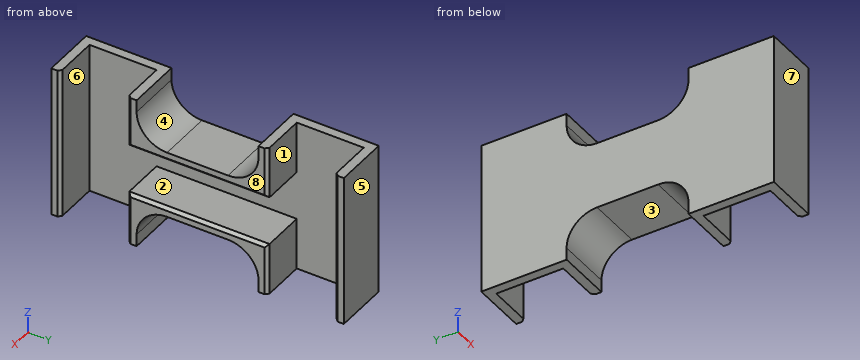
```python
from build123d import *

# Parameters (mm, degrees)
SKETCH1_W           = 22
SKETCH1_H           = 40
SKETCH1_W_2         = 50
SKETCH1_H_2         = 28
BOSS_EXTRUDE1_DEPTH = 18
SKETCH2_W           = 16
SKETCH2_H           = 46
CUT_EXTRUDE1_DEPTH  = 15
FILLET1_R           = 10
CHAMFER1_SIZE       = 1


with BuildPart() as part:
    # Sketch1 → Boss-Extrude1 (new body)
    with BuildSketch(Plane(origin=(0, 0, 0), x_dir=(0, 0, -1), z_dir=(1, 0, 0))):
        Polygon((0, 68), (14, 68), (36, 68), (50, 68), (50, 96), (0, 96), align=None)
        with Locations((25, 48)):
            Rectangle(SKETCH1_W, SKETCH1_H)
        with Locations((25, 14)):
            Rectangle(SKETCH1_W_2, SKETCH1_H_2)
    extrude(amount=BOSS_EXTRUDE1_DEPTH)

    # Sketch2 → Cut-Extrude1 (cut)
    with BuildSketch(Plane(origin=(18, 0, 0), x_dir=(0, 0, -1), z_dir=(1, 0, 0))):
        Polygon((50, 93), (0, 93), (0, 71), (17, 71), (33, 71), (50, 71), align=None)
        with Locations((25, 48)):
            Rectangle(SKETCH2_W, SKETCH2_H)
        Polygon((33, 25), (17, 25), (0, 25), (0, 3), (50, 3), (50, 25), align=None)
    extrude(amount=-CUT_EXTRUDE1_DEPTH, mode=Mode.SUBTRACT)

    # Fillet1
    fillet1_edges = [part.edges().sort_by_distance(p)[0] for p in [
        (9, 68, -36),
        (9, 28, -36),
        (9, 28, -14),
        (9, 68, -14),
    ]]
    fillet(fillet1_edges, radius=FILLET1_R)

    # Chamfer1
    chamfer1_edges = [part.edges().sort_by_distance(p)[0] for p in [
        (18, 93, -25),
        (18, 48, -33),
        (18, 25, -41.5),
        (18, 25, -8.5),
        (18, 71, -8.5),
        (18, 48, -17),
        (18, 3, -25),
        (18, 71, -41.5),
    ]]
    chamfer(chamfer1_edges, length=CHAMFER1_SIZE)


solid = part.part
```
Check sheet for the modelled part. Datum: model origin and axes. Units: mm. Face numbers are marked on the shaded views. A direction names the side the tool comes from. Round coordinates to 2 decimals unless told otherwise and drop trailing zeros. Order: outer loops, then holes, each group sorted by start corner. A loop starts at its lowest first (then second) coordinate and runs counter-clockwise, first axis right, second up.
1) Go/stop test with flat-tipped pins: pin 1 Ø1.5 at (y, z) = (69.5, -27.5) entering from +X; pin 2 Ø5 at (x, y) = (13, 64) entering from +Z; pin 3 Ø8 at (y, z) = (52, -42) entering from -X; pin 4 Ø5.5 at (x, y) = (12, 52) entering from +Z. Record where each tip stops, or that it passes through.
2) Scan lines: line 1 (Z direction, x = 16.5, y = 43); line 2 (Y direction, x = 13.75, z = -32); line 3 (Y direction, x = 16.25, z = -40). Record each from-to range of solid material in increasing order.
3) Tool access check on the marked faces 1, 2, 3 and 4. Record the directions out of +Z, -Z, +X, -X, +Y, -Y that give a thin tool (end or side, any length) a straight path to the whole face; none if there is none.
4) Section check B-B (z = -40.5). Record the boundary of the cut face in (x, y), and give its area (3 significant figures).
5) Section check C-C (z = -15). Record the boundary of the cut face in (x, y), and give its area (3 significant figures).
6) Section check D-D (y = 63.5). Record the boundary of the cut face in (x, z), and give its area (3 significant figures).
7) Mould release check, pull along Y, two halves, no side actions. Record for the marked faces 5, 6, 7 and 8: +Y half, -Y half, draft (parallel to the pull), parting line (faces both ways), or undercut.
8) Section check A-A (x = 5). Record the boundary of the cut face in (y, z).
Result:
1. pin 1: stops at x = 3
1. pin 2: stops at z = -9.27
1. pin 3: passes through
1. pin 4: stops at z = -14
2. line 1: z = -36 to -33, -17 to -14
2. line 2: y = 0 to 3, 93 to 96
2. line 3: y = 0 to 3, 25 to 30, 66 to 71, 93 to 96
3. face 1: +Z, -Z, +X
3. face 2: +X
3. face 3: -Z, +X, -X
3. face 4: +Z, +X, -X
4. outline: (0, 0) - (18, 0) - (18, 2) - (17, 3) - (3, 3) - (3, 25) - (17, 25) - (18, 26) - (18, 29.65) - (0, 29.65) - close; (0, 66.35) - (18, 66.35) - (18, 70) - (17, 71) - (3, 71) - (3, 93) - (17, 93) - (18, 94) - (18, 96) - (0, 96) - close
4. area: 405 mm2
5. outline: (0, 0) - (18, 0) - (18, 2) - (17, 3) - (3, 3) - (3, 25) - (17, 25) - (18, 26) - (18, 70) - (17, 71) - (3, 71) - (3, 93) - (17, 93) - (18, 94) - (18, 96) - (0, 96) - close
5. area: 1,070 mm2
6. outline: (0, -37.65) - (18, -37.65) - (18, -34) - (17, -33) - (3, -33) - (3, -17) - (17, -17) - (18, -16) - (18, -12.35) - (0, -12.35) - close
6. area: 214 mm2
7. face 5: +Y half
7. face 6: undercut
7. face 7: -Y half
7. face 8: draft
8. outline: (0, -50) - (3, -50) - (3, 0) - (0, 0) - close; (25, -50) - (28, -50) - (28, -46) arc R10 cw to (38, -36) - (58, -36) arc R10 cw to (68, -46) - (68, -50) - (71, -50) - (71, -33) - (25, -33) - close; (25, -17) - (71, -17) - (71, 0) - (68, 0) - (68, -4) arc R10 cw to (58, -14) - (38, -14) arc R10 cw to (28, -4) - (28, 0) - (25, 0) - close; (93, -50) - (96, -50) - (96, 0) - (93, 0) - close
